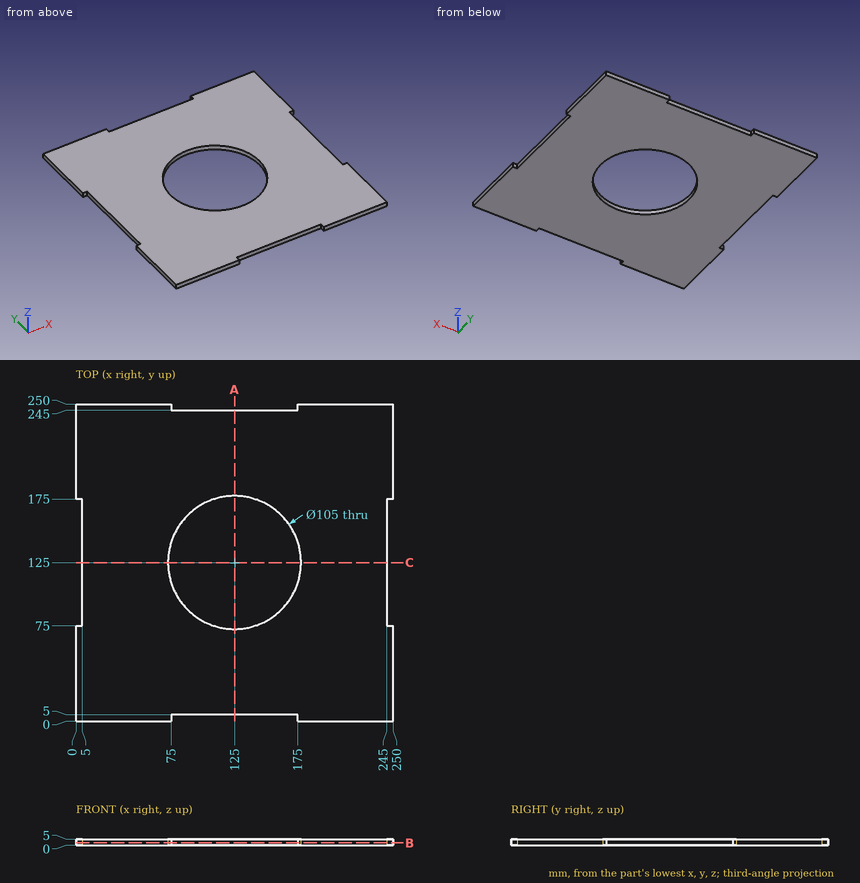
Design review of the part shown in the three views and the two pictorial views. Dimensions are in mm from the part's minimum x, y and z. Round coordinates to 2 decimals unless told otherwise and drop trailing zeros. Order: outer loops, then holes, each group sorted by start corner. A loop starts at its lowest first (then second) coordinate and runs counter-clockwise, first axis right, second up. Notation, with made-up numbers: (44, 60) -> (65, 60) arc R26 ccw to (65, 77) -> close; hole circle Ø9 at (-12, 40.25). An arc over 180 degrees is marked (long way). Write item = value, one per line. Start each with the question number.
1) Take a section at B-B on z = 1.95. State the section outline as (x, y) points, plus the area to 3 significant figures.
2) Insertion check: pin 1 (1.5 mm diameter, centred on x = 147, z = 1.5, fed in from -Y). The pin has a flat end and moves straight along its axis. Give the tip position at first contact, or say it passes through.
3) Take a section at A-A on x = 125. State the section outline as (y, z) points.
4) To check wall thickness, follow line 1 (Y direction, x = 125, z = 3.8); line 2 (Y direction, x = 166, z = 2.45); line 3 (X direction, y = 173, z = 0.65). State the ranges of each line that lie inside material, in increasing order. Write a range as from..to.
Verdict:
q1.outline = (0, 0) -> (75, 0) -> (75, 5) -> (175, 5) -> (175, 0) -> (250, 0) -> (250, 75) -> (245, 75) -> (245, 175) -> (250, 175) -> (250, 250) -> (175, 250) -> (175, 245) -> (75, 245) -> (75, 250) -> (0, 250) -> (0, 175) -> (5, 175) -> (5, 75) -> (0, 75) -> close; hole circle Ø105 at (125, 125)
q1.area = 51,800 mm2
q2.pin_1 = 5
q3.outline = (5, 0) -> (72.5, 0) -> (72.5, 5) -> (5, 5) -> close; (177.5, 0) -> (245, 0) -> (245, 5) -> (177.5, 5) -> close
q4.line_1 = 5..72.5, 177.5..245
q4.line_2 = 5..92.21, 157.79..245
q4.line_3 = 5..103.73, 146.27..245
